Geometry check sheet. Reference: the model listing, model coordinates, mm. A direction names the side the tool comes from. Give positions to 0.01 mm unless a question says otherwise; leave off trailing zeros. Order: outer loops, then holes, each group sorted by start corner. A loop starts at its lowest first (then second) coordinate and runs counter-clockwise, first axis right, second up.
from build123d import *

# Parameters (mm, degrees)
F1_DEPTH = 6.35
F2_W     = 5.35
F2_H     = 5.35
F3_DEPTH = 6.35
F4_W     = 37
F4_H     = 37
F5_DEPTH = 25


# Not quite as in the source:
# - a length typed as a fraction of an inch, garbled in the dataset ("3 / 203.2 mm" for 3/8 in), is restored


with BuildPart() as f1:
    # F0 (on Front) → F1 (new body)
    with BuildSketch(Plane.XZ):
        Polygon((17.5, -30.3108891325), (35, 0), (17.5, 30.3108891325), (-17.5, 30.3108891325), (-35, 0), (-17.5, -30.3108891325), align=None)
    extrude(amount=F1_DEPTH)

    # F2 (on face) → F3 (join)
    with BuildSketch(Plane.XZ.offset(6.35)):
        with Locations((0, 32.9858891325)):
            Rectangle(F2_W, F2_H)
        with Locations((0, -32.9858891325)):
            Rectangle(F2_W, F2_H)
        Polygon((29.5457359102, 20.1470625214), (24.9125, 17.4720625214), (27.5875, 12.8388266111), (32.2207359102, 15.5138266111), align=None)
        Polygon((-32.2207359102, 15.5138266111), (-27.5875, 12.8388266111), (-24.9125, 17.4720625214), (-29.5457359102, 20.1470625214), align=None)
        Polygon((-24.9125, -17.4720625214), (-27.5875, -12.8388266111), (-32.2207359102, -15.5138266111), (-29.5457359102, -20.1470625214), align=None)
        Polygon((27.5875, -12.8388266111), (24.9125, -17.4720625214), (29.5457359102, -20.1470625214), (32.2207359102, -15.5138266111), align=None)
    extrude(amount=-F3_DEPTH)

    # F4 (on face) → F5 (cut)
    with BuildSketch(Plane.XZ.offset(6.35)):
        Rectangle(F4_W, F4_H)
    extrude(amount=-F5_DEPTH, mode=Mode.SUBTRACT)


solid = f1.part
Item 1: Sectioned sample at D-D (x = 23). Enter the section's corners in (y, z).
Reported:
outline: (-6.35, -20.78) - (0, -20.78) - (0, 20.78) - (-6.35, 20.78) - close
Item 2: Sectioned sample at B-B (x = 4.5). Enter the section's corners in (y, z), and give its area (3 significant figures).
Reported:
outline: (-6.35, -30.31) - (0, -30.31) - (0, -18.5) - (-6.35, -18.5) - close; (-6.35, 18.5) - (0, 18.5) - (0, 30.31) - (-6.35, 30.31) - close
area: 150 mm2
Item 3: Draft check along Z on faces 1 (the flat face through (-21.154, -3.131, 23.981)), 2 (the flat face through (0, -3, 18.5)), 3 (the flat face through (-2.675, -3, 33)). Enter one of: released by +Z, released by -Z, zero draft, split by the parting line, or undercut.
Reported:
face 1: released by +Z
face 2: undercut
face 3: zero draft
Item 4: Sectioned sample at C-C (z = -4). Enter the section's corners in (x, y).
Reported:
outline: (-32.69, -6.35) - (-18.5, -6.35) - (-18.5, 0) - (-32.69, 0) - close; (18.5, -6.35) - (32.69, -6.35) - (32.69, 0) - (18.5, 0) - close
Item 5: Set-up check for faces 4 (the flat face through (2.675, -3, -33)), 5 (the flat face through (29.937, -3.219, -14.195)), 6 (the flat face through (-31.346, -3.131, -6.33)), 7 (the flat face through (-27.197, -3.219, 18.791)): record each of +Z, -Z, +X, -X, +Y, -Y from which the full face is reachable in a straight line by a thin tool's end or side.
Reported:
face 4: -Z, +X, +Y, -Y
face 5: +X, +Y, -Y
face 6: -X, +Y, -Y
face 7: +Z, +Y, -Y
Item 6: Gauge pin test, flat ends, axial feed: pin 1 (3 mm diameter, centred on y = -3.5, z = -10.5, fed in from +X); pin 2 (1.9 mm diameter, centred on x = 7, y = -2, fed in from -Z); pin 3 (3 mm diameter, centred on x = -13, y = -2, fed in from +Z). Record the tip position at first contact, or that the pin passes through.
Reported:
pin 1: stops at x = 29.8
pin 2: stops at z = -30.31
pin 3: stops at z = 30.31
Item 7: Scan lines: L1, parallel to Z at x = -9.5, y = -4; L2, parallel to Z at x = 30.5, y = -5.75; L3, parallel to Z at x = 28, y = -1.25. Record each from-to range of solid material in increasing order.
Reported:
L1: z = -30.31 to -18.5, 18.5 to 30.31
L2: z = -18.49 to -14.52, -7.79 to 7.79, 14.52 to 18.49
L3: z = -19.25 to -13.08, -12.12 to 12.12, 13.08 to 19.25
